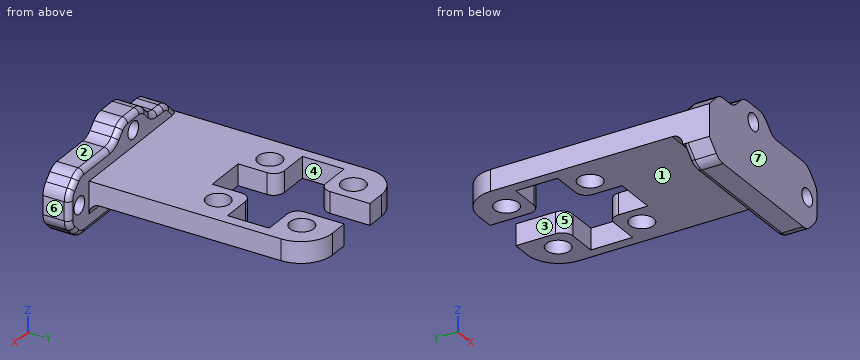
Autodesk Inventor part; units mm, degrees
ref_plane "YZ Plane" through (0, 0, 0) normal (1, 0, 0) x (0, 1, 0)
ref_plane "XZ Plane" through (0, 0, 0) normal (0, 1, 0) x (-1, 0, 0)
ref_plane "XY Plane" through (0, 0, 0) normal (0, 0, 1) x (1, 0, 0)
sketch "Sketch1" plane through (0, 0, 0) normal (0, 0, 1) x (1, 0, 0)
  line L0 (0, 0) -> (26.86, 0)
  line L1 (26.86, 0) -> (26.86, 47.18)
  line L2 (26.86, 47.18) -> (0, 47.18)
  line L3 (0, 47.18) -> (0, 0)
  line L4 (2, 38.68) -> (8.5, 38.68)
  line L5 (8.5, 38.68) -> (8.5, 45.18)
  line L6 (8.5, 45.18) -> (18.36, 45.18)
  line L7 (18.36, 45.18) -> (18.36, 38.68)
  line L8 (18.36, 38.68) -> (24.86, 38.68)
  line L9 (24.86, 38.68) -> (24.86, 28.82)
  line L10 (24.86, 28.82) -> (18.36, 28.82)
  line L11 (18.36, 28.82) -> (18.36, 22.32)
  line L12 (18.36, 22.32) -> (8.5, 22.32)
  line L13 (8.5, 22.32) -> (8.5, 28.82)
  line L14 (2, 28.82) -> (2, 38.68)
  line L15 (2, 28.82) -> (8.5, 28.82)
  line L16 (2, 33.75) -> (24.86, 33.75) construction
  line L17 (13.43, 47.18) -> (13.43, 0) construction
  circle A0 centre (5.556, 41.624) radius 2.25
  circle A1 centre (5.556, 25.876) radius 2.25
  circle A2 centre (21.304, 25.876) radius 2.25
  circle A3 centre (21.304, 41.624) radius 2.25
  line L18 (8.5, 45.18) -> (8.5, 47.18)
  line L19 (18.36, 45.18) -> (18.36, 47.18)
  line L20 (5.556, 41.624) -> (21.304, 41.624)
  line L21 (21.304, 41.624) -> (21.304, 25.876)
  line L22 (21.304, 25.876) -> (5.556, 25.876)
  line L23 (5.556, 25.876) -> (5.556, 41.624)
  line L24 (26.86, 47.18) -> (17.36, 47.18)
  line L25 (17.36, 47.18) -> (17.36, 37.68)
  line L26 (17.36, 37.68) -> (26.86, 37.68)
  line L27 (26.86, 37.68) -> (26.86, 47.18)
  line L28 (0, 47.18) -> (9.5, 47.18)
  line L29 (9.5, 47.18) -> (9.5, 37.68)
  line L30 (9.5, 37.68) -> (0, 37.68)
  line L31 (0, 37.68) -> (0, 47.18)
  line L32 (0, 20.8011) -> (9.5, 20.8011)
  line L33 (9.5, 20.8011) -> (9.5, 29.82)
  line L34 (9.5, 29.82) -> (0, 29.82)
  line L35 (0, 29.82) -> (0, 20.8011)
  line L36 (26.86, 20.8011) -> (17.36, 20.8011)
  line L37 (17.36, 20.8011) -> (17.36, 29.82)
  line L38 (17.36, 29.82) -> (26.86, 29.82)
  line L39 (26.86, 29.82) -> (26.86, 20.8011)
  point P0 (13.43, 33.75)
  point P1 (5.25, 38.68)
  point P2 (9.5, 22.32)
  point P3 (2, 29.82)
  point P4 (5.556, 28.82)
  point P5 (5.556, 28.126)
  point P6 (7.806, 25.876)
  point P7 (8.5, 25.876)
  point P8 (17.36, 22.32)
  point P9 (18.36, 25.876)
  point P10 (19.054, 25.876)
  point P11 (21.304, 28.126)
  point P12 (21.304, 28.82)
  point P13 (24.86, 29.82)
  point P14 (24.86, 37.68)
  point P15 (21.304, 38.68)
  point P16 (21.304, 39.374)
  point P17 (19.054, 41.624)
  point P18 (18.36, 41.624)
  point P19 (8.5, 41.624)
  point P20 (7.806, 41.624)
  point P21 (5.556, 39.374)
  point P22 (5.556, 38.68)
  point P23 (2, 37.68)
  dimension "d0" = 47.18
  dimension "d1" = 26.86
  dimension "d2" = 6.5
  dimension "d3" = 22.86
  dimension "d4" = 2
  dimension "d5" = 4.5
  dimension "d6" = 2.944
  dimension "d7" = 2.944
  dimension "d19" = 15.748
  dimension "d20" = 15.748
  dimension "d21" = 1
  dimension "d22" = 1
  dimension "d23" = 1
  dimension "d24" = 1
extrude "Extrusion1" add sketch "Sketch1" along normal blind 6 contours L3 L32 L33 L12 L37 L36 L1 L0 | L3 L34 L14 L15 L23 A1 L22 L13 L12 L33 L32 | L36 L37 L12 L11 L22 A2 L21 L10 L9 L38 L1 | L3 L30 L14 L34 | L38 L9 L26 L1 | L3 L2 L18 L5 L20 A0 L23 L4 L14 L30 | L26 L9 L8 L21 A3 L20 L7 L19 L2 L1 | L15 L13 L22 A1 L23 | L21 A2 L22 L11 L10 | L23 A0 L20 L5 L4 | L8 L7 L20 A3 L21
fillet "Fillet1" radius 2 4 edges at (8.5, 28.82, 3) (18.36, 28.82, 3) (8.5, 38.68, 3) (18.36, 38.68, 3)
fillet "Fillet2" radius 6 2 edges at (0, 47.18, 3) (26.86, 47.18, 3)
sketch "Sketch2" plane through (0, 0, 6) normal (0, 0, 1) x (1, 0, 0)
  line L0 (8.5, 45.18) -> (18.36, 45.18)
  line L1 (24.86, 38.68) -> (24.86, 28.82)
  line L2 (18.36, 22.32) -> (8.5, 22.32)
  line L3 (2, 28.82) -> (2, 38.68)
  circle A0 centre (13.43, 33.75) radius 11.43
  point P0 (0, 0)
sketch "Sketch3" plane through (0, 0, 0) normal (0, -1, 0) x (1, 0, 0)
  line L0 (0, 0) -> (26.86, 0)
  line L1 (26.86, 0) -> (26.86, 6)
  line L2 (0, 6) -> (26.86, 6)
  line L3 (0, 0) -> (0, 6) construction
  line L4 (32.86, 6) -> (32.86, 0) construction
  line L5 (32.86, 0) -> (-6, 0) construction
  line L6 (0, 6) -> (26.86, 6) construction
  line L7 (0, 0) -> (26.86, 0) construction
  line L8 (13.43, 6) -> (13.43, 0) construction
  line L9 (13.43, 6) -> (13.43, 0) construction
  circle A0 centre (29.86, 3) radius 1.625
  line L10 (26.86, 6) -> (32.86, 0) construction
  circle A1 centre (13.43, 9) radius 1.625
  line L11 (29.86, -3) -> (32.86, 0) construction
  line L12 (29.86, 9) -> (32.86, 6) construction
  line L13 (0, 0) -> (0, 6) construction
  line L14 (0, 6) -> (0, 0) construction
  line L15 (26.86, 0) -> (26.86, 6) construction
  line L16 (26.86, 6) -> (26.86, 0) construction
  line L17 (0, 0) -> (0, 6) construction
  line L18 (0, 6) -> (3, 9) construction
  line L19 (3, 9) -> (7.43, 9)
  line L20 (7.43, 9) -> (10.43, 12)
  line L21 (10.43, 12) -> (16.43, 12)
  line L22 (16.43, 12) -> (19.43, 9)
  line L23 (19.43, 9) -> (29.86, 9)
  line L24 (26.86, 6) -> (26.86, 0) construction
  line L25 (13.43, 12) -> (13.43, 6) construction
  line L26 (7.43, 9) -> (19.43, 9) construction
  line L27 (18.36, 6) -> (8.5, 6) construction
  line L28 (0, 0) -> (3, -3) construction
  line L29 (3, -3) -> (29.86, -3)
  line L30 (0, 3) -> (32.86, 3) construction
  circle A2 centre (13.43, -3) radius 1.625 construction
  line L31 (7.43, -3) -> (10.43, -6) construction
  line L32 (10.43, -6) -> (16.43, -6) construction
  line L33 (16.43, -6) -> (19.43, -3) construction
  line L34 (0, 0) -> (3, -3)
  line L35 (3, -3) -> (7.43, -3)
  line L36 (19.43, -3) -> (29.86, -3)
  line L37 (29.86, -3) -> (32.86, 0)
  line L38 (32.86, 0) -> (32.86, 6)
  line L39 (32.86, 6) -> (29.86, 9)
  line L40 (29.86, 9) -> (3, 9) construction
  line L41 (3, 9) -> (0, 6)
  point P0 (13.43, 3)
  point P1 (26.86, 3)
  dimension "d12" = 6
  dimension "d13" = 3.25
  dimension "d28" = 3
  dimension "d29" = 6
  dimension "d30" = 6
  dimension "d31" = 135
  dimension "d32" = 3.25
  dimension "d33" = 3
  dimension "d36" = 6
extrude "Extrusion2" add sketch "Sketch3" against normal blind 5
extrude "Extrusion3" add sketch "Sketch1" along normal blind 6 contours L34 L23 L15 L14 | L12 L13 L22 L33 | L9 L10 L21 L38 | L37 L22 L11 L12 | L14 L4 L23 L30 | L34 L33 L22 L13 L15 L23 | L26 L21 L8 L9 | L21 L10 L11 L22 L37 L38 | L2 L29 L6 L18 | L23 L4 L5 L20 L29 L30 | L15 L13 L22 A1 L23 | L19 L6 L25 L2 | L26 L25 L20 L7 L8 L21 | L21 A2 L22 L11 L10 | L6 L29 L20 L5 | L23 A0 L20 L5 L4 | L7 L20 L25 L6 | L8 L7 L20 A3 L21
fillet "Fillet4" radius 2 4 edges at (9.5, 37.68, 3) (17.36, 37.68, 3) (9.5, 29.82, 3) (17.36, 29.82, 3)
fillet "Fillet9" radius 3 10 edges at (3, 2.5, 9) (7.43, 2.5, 9) (10.43, 2.5, 12) (16.43, 2.5, 12) (19.43, 2.5, 9) (29.86, 2.5, 9) (32.86, 2.5, 6) (32.86, 2.5, 0) (29.86, 2.5, -3) (3, 2.5, -3)
fillet "Fillet10" radius 1 21 edges at (3.0946, 5, -2.7716) (1.0607, 5, -1.0607) (29.7654, 5, -2.7716) (31.36, 5, -1.5) (32.6316, 5, 0.0946) (32.86, 5, 3) (32.6316, 5, 5.9054) (31.36, 5, 7.5) (29.7654, 5, 8.7716) (24.645, 5, 9) (19.5246, 5, 9.2284) (17.93, 5, 10.5) (16.3354, 5, 11.7716) (13.43, 5, 12) (10.5246, 5, 11.7716) (8.93, 5, 10.5) (7.3354, 5, 9.2284) (5.215, 5, 9) (3.0946, 5, 8.7716) (1.0607, 5, 7.0607) (16.43, 5, -3)
sketch "Sketch4" plane through (0, 0, 0) normal (0, 0, -1) x (-1, 0, 0)
  line L0 (-33.4061, 50.4352) -> (8.6296, 50.4352)
  line L1 (8.6296, 50.4352) -> (8.6296, 5)
  line L2 (8.6296, 5) -> (-33.4061, 5)
  line L3 (-33.4061, 5) -> (-33.4061, 50.4352)
  line L4 (-4.2426, 5) -> (-28.6174, 5)
  point P0 (0, 0)
extrude "Extrusion4" cut sketch "Sketch4" against normal blind 2
fillet "Fillet11" radius 2 1 edges at (13.43, 5, 2)
equation "\"d29\" = 2 * d28"
equation "\"d30\" = d29"
equation "\"d32\" = d13"
properties part number "as5600mount_2"
Source: CAD feature listing. Evaluate the final solid. Frame: model axes, mm. Face numbers are marked on the shaded views. A direction names the side the tool comes from. Coordinates: 2 decimals unless noted, no trailing zeros. Write each loop counter-clockwise with the first axis right and the second up, starting at its lowest first coordinate (ties: lowest second). Pieces come first, ordered by that corner, then holes. Notation, with made-up numbers: (33, 5) - (78, 5) arc R23 cw to (78, 15) - close; hole circle Ø5 at (-6.5, 60.25). An arc over 180 degrees is marked (long way). Answer as a JSON object with one key per item and string values.
Q1. Section query A-A, the plane x = 13.43. Output: boundary loops of the cut face in (y, z) (3 decimals).
Ans:
{"outline": "(0, -3) - (4, -3) arc R1 ccw to (5, -2) - (5, 0) arc R2 cw to (7, 2) - (22.32, 2) - (22.32, 6) - (5, 6) - (5, 7.375) - (0, 7.375) - close; (0, 10.625) - (5, 10.625) - (5, 11) arc R1 ccw to (4, 12) - (0, 12) - close"}
Q2. First-contact query: pin 1 Ø8 at (x, y) = (6.5, 31) entering from +Z; pin 2 Ø1 at (x, z) = (8, 8.5) entering from +Y; pin 3 Ø0.6 at (x, y) = (5.5, 2.5) entering from +Z; pin 4 Ø4 at (x, y) = (5.556, 41.624) entering from +Z. Flat tips, straight axial feed; report the tip coordinate or a pass-through.
Ans:
{"pin 1": "stops at z = 6", "pin 2": "stops at y = 5", "pin 3": "stops at z = 9", "pin 4": "passes through"}
Q3. Material intervals for line 1 (Z direction, x = 8, y = 43); line 2 (Y direction, x = 11.5, z = 6.75); line 3 (Z direction, x = 29, y = 3), sorted ascending. Write a range as [from, to].
Ans:
{"line 1": "z = [2, 6]", "line 2": "y = [0, 5]", "line 3": "z = [-2.98, 1.62], [4.38, 8.98]"}
Q4. Section query D-D, the plane y = 12.5. Output: boundary loops of the cut face in (x, z).
Ans:
{"outline": "(0, 2) - (26.86, 2) - (26.86, 6) - (0, 6) - close"}
Q5. Section query C-C, the plane z = 3. State how many separate pieces and enclosed holes the cut face has, plus the area to 3 significant figures.
Ans:
{"separate pieces": "2", "enclosed holes": "4", "area": "885 mm2"}
Q6. Draft query along X for the marked faces 5, 6 and 7. Return one class per face: released by +X, released by -X, zero draft, split by the parting line, or undercut.
Ans:
{"face 5": "undercut", "face 6": "released by +X", "face 7": "zero draft"}
Q7. Set-up query: the marked faces 1, 2, 3 and 4. Return all of +Z, -Z, +X, -X, +Y, -Y with unobstructed straight access to the full face (end or side cutting, diameter ignored); none if empty.
Ans:
{"face 1": "-Z, +X, -X, +Y", "face 2": "+Z, +X, +Y, -Y", "face 3": "+Z, -Z, +Y", "face 4": "+Z, -Z"}
Q8. Section query B-B, the plane y = 27. Output: boundary loops of the cut face in (x, z).
Ans:
{"outline": "(0, 2) - (3.61, 2) - (3.61, 6) - (0, 6) - close; (7.51, 2) - (9.5, 2) - (9.5, 6) - (7.51, 6) - close; (17.36, 2) - (19.35, 2) - (19.35, 6) - (17.36, 6) - close; (23.25, 2) - (26.86, 2) - (26.86, 6) - (23.25, 6) - close"}
